Input: dimensioned drawing with shaded views. Units: mm. Origin: part minimum x, y, z. Round coordinates to 2 decimals unless told otherwise and drop trailing zeros. Loops run counter-clockwise (first coordinate to the right, second up) from the corner with the lowest first, then second, coordinate; pieces in that order, holes last. Notation, with made-up numbers: (47, 7) -> (62, 7) arc R9 cw to (62, 18) -> close; hole circle Ø1 at (75, 38.5). An arc over 180 degrees is marked (long way). Answer as a JSON object with one key per item and string values.
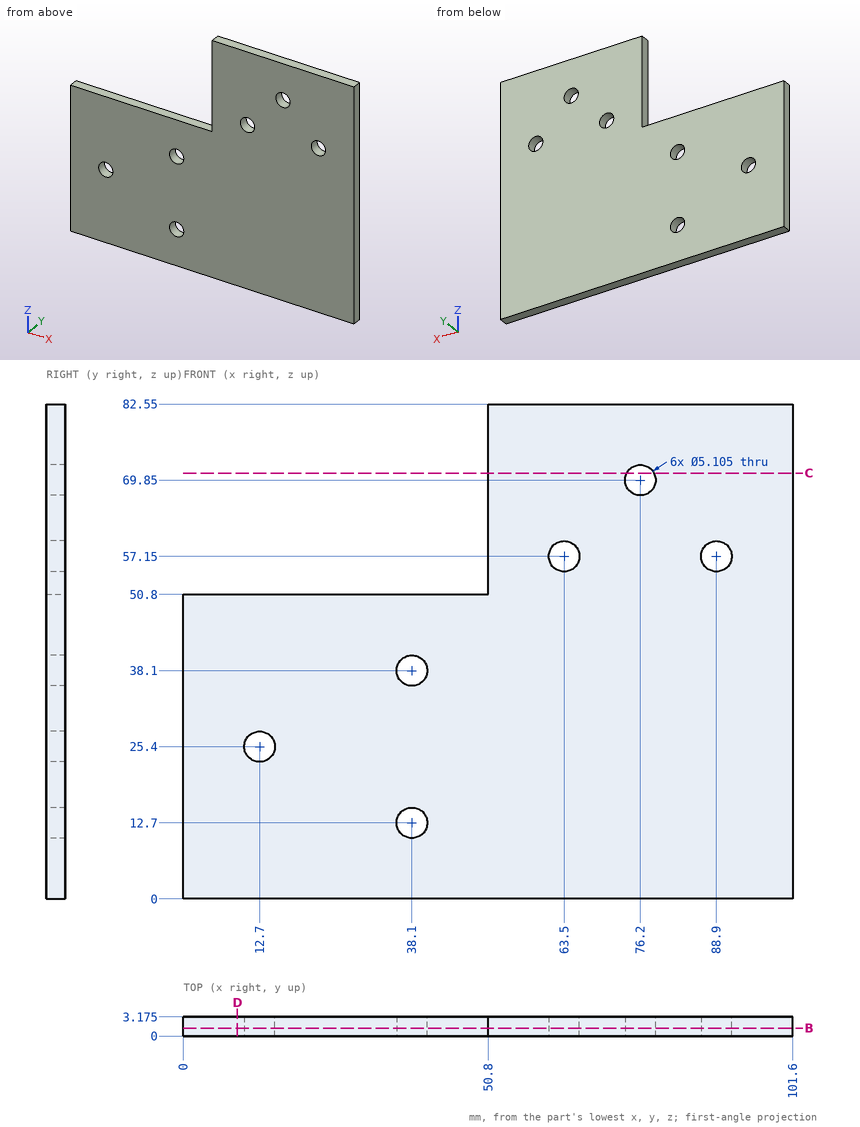
1) Ray query, probe 1 along Z at (x, y) = (12.7, 1.35); probe 2 along Z at (x, y) = (38.1, 2.2); probe 3 along Z at (x, y) = (88.9, 1). Return the intervals inside material, ascending.
Output:
{"probe 1": "z = 0 to 22.85, 27.95 to 50.8", "probe 2": "z = 0 to 10.15, 15.25 to 35.55, 40.65 to 50.8", "probe 3": "z = 0 to 54.6, 59.7 to 82.55"}
2) Section B-B, the plane y = 1.3. Count the separate pieces of the cut face and the enclosed holes in it, plus the area to 3 significant figures.
Output:
{"separate pieces": "1", "enclosed holes": "6", "area": "6,650 mm^2"}
3) Section D-D, the plane x = 9. Output: boundary loops of the cut face in (y, z) (1 decimal), plus the area to 3 significant figures.
Output:
{"outline": "(0, 0) -> (3.2, 0) -> (3.2, 50.8) -> (0, 50.8) -> close", "area": "161 mm^2"}
4) Contact query for flat-ended pins moving along their axis: P1, Ø4, axis at x = 38.1, z = 38.1, coming from the +Y side; P2, Ø1, axis at x = 25, y = 2.5, coming from the +Z side; P3, Ø1.6, axis at y = 1, z = 73, coming from the -X side. Output: stop coordinate, or through.
Output:
{"P1": "passes through", "P2": "stops at z = 50.8", "P3": "stops at x = 50.8"}
5) Section C-C, the plane z = 71. Output: boundary loops of the cut face in (x, y) (1 decimal).
Output:
{"outline": "(50.8, 0) -> (73.9, 0) -> (73.9, 3.2) -> (50.8, 3.2) -> close; (78.5, 0) -> (101.6, 0) -> (101.6, 3.2) -> (78.5, 3.2) -> close"}
